Read the model definition and answer for the solid it produces. Units are mm, in the model's axes. A direction names the side the tool comes from. Give positions to 0.01 mm unless a question says otherwise; leave off trailing zeros. Order: outer loops, then holes, each group sorted by start corner. A loop starts at its lowest first (then second) coordinate and runs counter-clockwise, first axis right, second up. Notation, with made-up numbers: (-6, 32.25) - (14, 32.25) arc R34 ccw to (14, 67.25) - close; hole circle Ø8 at (8, 72.25). An arc over 180 degrees is marked (long way). Answer as CSV lines item,"result". Start each with the question number.
from build123d import *

# Parameters (mm, degrees)
SKETCH1_W           = 33.08
SKETCH1_H           = 33.08
SKETCH1_W_2         = 28
SKETCH1_H_2         = 28
EXTRUDE_THIN1_DEPTH = 25.4
CIRPATTERN1_COUNT   = 4
SKETCH1_3_W         = 28
SKETCH1_3_H         = 28
SKETCH1_3_W_2       = 20
SKETCH1_3_H_2       = 20
BOSS_EXTRUDE1_DEPTH = 1.27
FILLET1_R           = 3.81


with BuildPart() as part:
    # Sketch1 → Extrude-Thin1 (new body)
    with BuildSketch(Plane(origin=(0, 0, 0), x_dir=(1, 0, 0), z_dir=(0, 1, 0))):
        with Locations((14, 14)):
            Rectangle(SKETCH1_W, SKETCH1_H)
        with Locations((14, 14)):
            Rectangle(SKETCH1_W_2, SKETCH1_H_2, mode=Mode.SUBTRACT)
    extrude(amount=EXTRUDE_THIN1_DEPTH)

    # Sketch9 → Tap Drill for 1/4-20 Tap2 (revolve, cut)
    with BuildSketch(Plane(origin=(14, 12.7, 2.54), x_dir=(0, -1, 0), z_dir=(1, 0, 0))):
        Polygon((0, 0), (0, 9.153816902), (2.5527, 7.62), (2.5527, 0), align=None)
    tap_drill_for_1_4_20_tap2 = revolve(axis=Axis((14, 12.7, 8.89), (0, 0, -1)), mode=Mode.SUBTRACT)

    # CirPattern1: Tap Drill for 1/4-20 Tap2 ×4 about axis
    cirpattern1_axis = Axis((14, -1.27, -14), (0, 1, 0))
    for i in range(1, CIRPATTERN1_COUNT):
        add(tap_drill_for_1_4_20_tap2.rotate(cirpattern1_axis, i * 360 / CIRPATTERN1_COUNT), mode=Mode.SUBTRACT)

    # Sketch1<3> → Boss-Extrude1 (add)
    with BuildSketch(Plane(origin=(0, 0, 0), x_dir=(1, 0, 0), z_dir=(0, 1, 0))):
        with Locations((14, 14)):
            Rectangle(SKETCH1_3_W, SKETCH1_3_H)
        with Locations((14, 14)):
            Rectangle(SKETCH1_3_W_2, SKETCH1_3_H_2, mode=Mode.SUBTRACT)
    extrude(amount=BOSS_EXTRUDE1_DEPTH)

    # Fillet1
    fillet1_edges = [part.edges().sort_by_distance(p)[0] for p in [
        (0, 1.27, -14),
        (14, 1.27, 0),
        (28, 1.27, -14),
        (14, 1.27, -28),
    ]]
    fillet(fillet1_edges, radius=FILLET1_R)


solid = part.part
(1) Section C-C, the plane z = -9.5 is taken. Write down the section's boundary in (x, y), and give its area (3 significant figures).
(2) Straight lines are drawn through the part: line 1 (X direction, y = 6.5, z = -27); line 2 (X direction, y = 12.7, z = -28.85); line 3 (Z direction, x = 2, y = 14.25). For each, find the intervals that lie inside material, in ascending order. Write a range as [from, to].
(3) Determine the mould class of faces 4 (the flat face through (13.8, 9.7, 2.54)), 5 (the flat face through (14, 0, -3)), 6 (the flat face through (24, 1, -14)) for opening direction Z: released by +Z, released by -Z, zero draft, split by the parting line, or undercut.
(4) Section D-D, the plane y = 16.25 is taken. Write down the section's boundary in (x, z), and give its area (3 significant figures).
(5) Section A-A, the plane z = -14 is taken. Write down the section's boundary in (x, y), and give its area (3 significant figures).
(6) Section B-B, the plane x = 7 is taken. Write down the section's boundary in (y, z).
(7) Flat-ended cylindrical pins translate along their axes: pin 1 Ø4 at (x, y) = (14, 12.7) entering from -Z; pin 2 Ø2 at (x, z) = (25.5, -23) entering from +Y. Find the tip coordinate at first contact, or state that the pin passes through.
(8) Which of the six approach directions +Z, -Z, +X, -X, +Y, -Y give full straight-line access (tool end or side, diameter ignored) to faces 1 (the cylindrical face through (16.152, 11.328, -29.288)), 2 (the flat face through (28, 17, -14)), 3 (the flat face through (14, 1, -4))?
Checks:
1,outline,"(-2.54, 0) - (4, 0) - (4, 1.27) - (3.81, 1.27) arc R3.81 cw to (0, 5.08) - (0, 25.4) - (-2.54, 25.4) - close; (24, 0) - (30.54, 0) - (30.54, 25.4) - (28, 25.4) - (28, 5.08) arc R3.81 cw to (24.19, 1.27) - (24, 1.27) - close"
1,area,"145 mm²"
2,line 1,"x = [-2.54, 0], [28, 30.54]"
2,line 2,"x = [-2.54, 11.45], [16.55, 30.54]"
2,line 3,"z = [-30.54, -28], [0, 2.54]"
3,face 4,"released by +Z"
3,face 5,"zero draft"
3,face 6,"undercut"
4,outline,"(-2.54, -30.54) - (30.54, -30.54) - (30.54, 2.54) - (-2.54, 2.54) - close; hole (0, -28) - (28, -28) - (28, 0) - (0, 0) - close"
4,area,"310 mm²"
5,outline,"(-2.54, 0) - (4, 0) - (4, 1.27) - (3.81, 1.27) arc R3.81 cw to (0, 5.08) - (0, 10.15) - (-2.54, 10.15) - close; (-2.54, 15.25) - (0, 15.25) - (0, 25.4) - (-2.54, 25.4) - close; (24, 0) - (30.54, 0) - (30.54, 10.15) - (28, 10.15) - (28, 5.08) arc R3.81 cw to (24.19, 1.27) - (24, 1.27) - close; (28, 15.25) - (30.54, 15.25) - (30.54, 25.4) - (28, 25.4) - close"
5,area,"119 mm²"
6,outline,"(0, -30.54) - (25.4, -30.54) - (25.4, -28) - (5.08, -28) arc R3.81 cw to (1.27, -24.19) - (1.27, -24) - (0, -24) - close; (0, -4) - (1.27, -4) - (1.27, -3.81) arc R3.81 cw to (5.08, 0) - (25.4, 0) - (25.4, 2.54) - (0, 2.54) - close"
7,pin 1,"passes through"
7,pin 2,"stops at y = 2.05"
8,face 1,"+Z, -Z"
8,face 2,"+Y"
8,face 3,"+Y, -Y"
